from build123d import *

# Parameters (mm, degrees)
F0_W      = 200
F0_H      = 75
F1_DEPTH  = 200
F2_W      = 200
F2_H      = 15
F3_DEPTH  = 125
F4_W      = 68
F4_H      = 10
F5_DEPTH  = 120
F7_DEPTH  = 15
F8_R      = 3
F9_DEPTH  = 5
F10_R     = 20.5
F11_DEPTH = 25


with BuildPart() as f1:
    # F0 (on Top) → F1 (new body)
    with BuildSketch(Plane.XY):
        Polygon((-100, -75), (-100, 0), (-300, 0), (-300, -200), (-100, -200), align=None)
        Polygon((300, 0), (100, 0), (100, -75), (100, -200), (300, -200), align=None)
        with Locations((0, -37.5)):
            Rectangle(F0_W, F0_H)
    extrude(amount=F1_DEPTH)

    # F2 (on face) → F3 (join)
    with BuildSketch(Plane.XZ.offset(75)):
        with Locations((0, 192.5)):
            Rectangle(F2_W, F2_H)
    extrude(amount=F3_DEPTH)

    # F4 (on face) → F5 (join)
    with BuildSketch(Plane.XY.offset(200)):
        with Locations((0, -80)):
            Rectangle(F4_W, F4_H)
    extrude(amount=F5_DEPTH)

    # F6 (on face) → F7 (cut, through all)
    with BuildSketch(Plane.XY.offset(200)):
        with BuildLine():
            add(Edge.make_bspline(
                [(5, -92.05), (5, -87.719873), (-2.5, -89.884936), (-10, -92.05), (-2.5, -94.215064), (5, -96.380127), (5, -92.05)],
                knots=[0, 0, 0, 2.094395, 2.094395, 4.18879, 4.18879, 6.283185, 6.283185, 6.283185], degree=2, weights=[1, 0.5, 1, 0.5, 1, 0.5, 1]))
        make_face()
    extrude(amount=-F7_DEPTH, mode=Mode.SUBTRACT)

    # F8 (on face) → F9 (cut)
    with BuildSketch(Plane.XZ.offset(75)):
        with Locations((0, 125)):
            Circle(F8_R)
    extrude(amount=-F9_DEPTH, mode=Mode.SUBTRACT)

    # F10 (on face) → F11 (cut)
    with BuildSketch(Plane.XY.offset(200)):
        with Locations((-200, -100)):
            Circle(F10_R)
        with Locations((200, -100)):
            Circle(F10_R)
    extrude(amount=-F11_DEPTH, mode=Mode.SUBTRACT)


solid = f1.part
For this review, take the finished solid that the model builds, in its own axes (mm). A direction names the side the tool comes from. Coordinates: 2 decimals unless noted, no trailing zeros. Write each loop counter-clockwise with the first axis right and the second up, starting at its lowest first coordinate (ties: lowest second). Pieces come first, ordered by that corner, then holes. Notation, with made-up numbers: (6, 84) -> (25, 84) arc R11 cw to (25, 95) -> close; hole circle Ø10 at (54.25, 10). An arc over 180 degrees is marked (long way). Write each question's results on one line, items separated by ' | '. Start each with the question number.
1) Consider section A-A (x = -16.5). Write out the cut boundary in (y, z).
2) For faces 1 (the face through (-4, -200, 190)), 2 (the face through (-300, -99, 99)), 3 (the face through (0, -85, 259)), 4 (the face through (100, -137, 91)), 5 (the face through (-220.48, -99.1, 187.68)), list the 3-axis set-ups (+Z, -Z, +X, -X, +Y, -Y) from which the entire face can be reached by the end or side of a thin tool; tool diameter is ignored.
3) Consider section B-B (z = 44). Write out the cut boundary in (x, y).
4) The part is to be moulded in two halves that separate along X. For faces 6 (the face through (300, -101, 99)), 7 (the face through (0, -75, 259)), 8 (the face through (-100, -138, 91)), say which applies: +X half, -X half, draft (parallel to the pull), parting line (faces both ways), or undercut.
5) Insertion check: pin 1 (6 mm diameter, centred on x = 200, y = -179, fed in from +Z); pin 2 (6.5 mm diameter, centred on x = -0.5, z = 124.5, fed in from -Y); pin 3 (3 mm diameter, centred on y = -79, z = 265, fed in from -X). Each pin has a flat end and moves straight along its axis. Give the tip position at first contact, or say it passes through.
6) Consider section D-D (x = 53). Write out the cut boundary in (y, z).
7) Wall thickness on L1, parallel to Y at x = 200, z = 182.5; L2, parallel to X at y = -173, z = 155.5; L3, parallel to Z at x = 0, y = -71.4: over which ranges is each line inside the solid? List them lowest first. Write a range as [from, to].
8) Consider section C-C (y = -128). Write out the cut boundary in (x, z).
Geometry says:
1) outline: (-200, 185) -> (-75, 185) -> (-75, 0) -> (0, 0) -> (0, 200) -> (-75, 200) -> (-75, 320) -> (-85, 320) -> (-85, 200) -> (-200, 200) -> close
2) face 1: +Z, -Z, +X, -X, -Y | face 2: +Z, -Z, -X, +Y, -Y | face 3: +Z, +X, -X, -Y | face 4: -Z, -Y | face 5: +Z
3) outline: (-300, -200) -> (-100, -200) -> (-100, -75) -> (100, -75) -> (100, -200) -> (300, -200) -> (300, 0) -> (-300, 0) -> close
4) face 6: +X half | face 7: draft | face 8: undercut
5) pin 1: z = 200 | pin 2: y = -75 | pin 3: x = -34
6) outline: (-200, 185) -> (-75, 185) -> (-75, 0) -> (0, 0) -> (0, 200) -> (-200, 200) -> close
7) L1: [-200, -120.5], [-79.5, 0] | L2: [-300, -100], [100, 300] | L3: [0, 122], [128, 200]
8) outline: (-300, 0) -> (-100, 0) -> (-100, 185) -> (100, 185) -> (100, 0) -> (300, 0) -> (300, 200) -> (-300, 200) -> close
